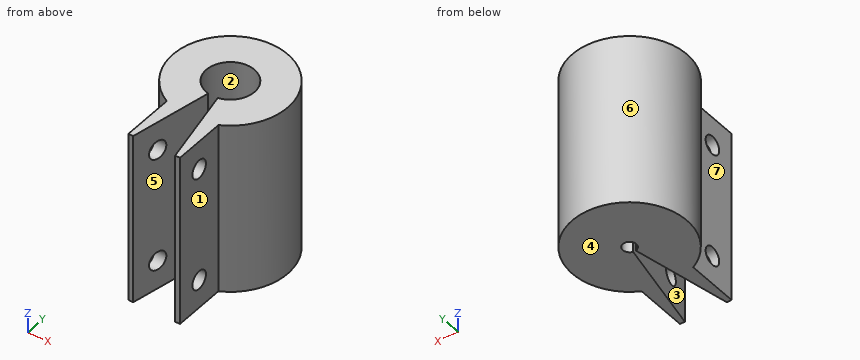
```python
from build123d import *

# Parameters (mm, degrees)
EXTRUDE_1_DEPTH     = 30
SKETCH_2_R          = 4.2
CUT_EXTRUDE_1_DEPTH = 15
SKETCH_3_R          = 1.175
CUT_EXTRUDE_2_DEPTH = 15
SKETCH_10_R         = 1.6
CUT_EXTRUDE_8_DEPTH = 38.871493237
CUT_EXTRUDE_9_DEPTH = 37.386810797


with BuildPart() as part:
    # ｽｹｯﾁ1 → ﾎﾞｽ - 押し出し1 (new body)
    with BuildSketch(Plane.XY):
        with BuildLine():
            Line((-4.5, -8.93028555), (-4.5, -18))
            Line((-4.5, -18), (4.5, -18))
            Line((4.5, -18), (4.5, -8.93028555))
            ThreePointArc((4.5, -8.93028555), (0, 10), (-4.5, -8.93028555))
        make_face()
    extrude(amount=EXTRUDE_1_DEPTH)

    # ｽｹｯﾁ2 → ｶｯﾄ - 押し出し1 (cut)
    with BuildSketch(Plane.XY.offset(30)):
        Circle(SKETCH_2_R)
    extrude(amount=-CUT_EXTRUDE_1_DEPTH, mode=Mode.SUBTRACT)

    # ｽｹｯﾁ3 → ｶｯﾄ - 押し出し2 (cut)
    with BuildSketch(Plane(origin=(0, 0, 0), x_dir=(-1, 0, 0), z_dir=(0, 0, -1))):
        Circle(SKETCH_3_R)
    extrude(amount=-CUT_EXTRUDE_2_DEPTH, mode=Mode.SUBTRACT)

    # ｽｹｯﾁ10 → ｶｯﾄ - 押し出し8 (cut, through all)
    with BuildSketch(Plane(origin=(4.5, 0, 0), x_dir=(0, 0, -1), z_dir=(1, 0, 0))):
        with Locations(Location((-25, -13.465142775, 0), (0, 0, 90))):
            Circle(SKETCH_10_R)
        with Locations(Location((-5, -13.465142775, 0), (0, 0, 90))):
            Circle(SKETCH_10_R)
    extrude(amount=-CUT_EXTRUDE_8_DEPTH, mode=Mode.SUBTRACT)

    # ｽｹｯﾁ4 → ｶｯﾄ - 押し出し9 (cut, through all)
    with BuildSketch(Plane.XY.offset(30)):
        with BuildLine():
            Line((-0.234043532, -1.151455003), (-3.658661061, -18))
            ThreePointArc((-3.658661061, -18), (0, -18.368064698), (3.658661061, -18))
            Line((3.658661061, -18), (0.234043532, -1.151455003))
            ThreePointArc((0.234043532, -1.151455003), (0, -1.175), (-0.234043532, -1.151455003))
        make_face()
    extrude(amount=-CUT_EXTRUDE_9_DEPTH, mode=Mode.SUBTRACT)


solid = part.part
```
The model under review builds one solid part; all positions refer to its coordinate system, in mm. Face numbers are marked on the shaded views. A direction names the side the tool comes from. Round coordinates to 2 decimals unless told otherwise and drop trailing zeros. Loops run counter-clockwise (first coordinate to the right, second up) from the corner with the lowest first, then second, coordinate; pieces in that order, holes last. Notation, with made-up numbers: (11, -12) -> (22, -12) arc R10 cw to (22, 4) -> close; hole circle Ø3 at (-6, -7). An arc over 180 degrees is marked (long way). Answer in a Markdown table with one row per item.
1) For pin 1 Ø10 at (y, z) = (-15.5, 20) entering from -X; pin 2 Ø6 at (x, y) = (-3, 6) entering from -Z; pin 3 Ø7.5 at (y, z) = (-13, 8.5) entering from +X; pin 4 Ø8 at (x, z) = (5, 21) entering from +Y, all flat-tipped, find the tip position at first contact; note any pin that passes through.
Taken from the geometry:
| item | result |
|---|---|
| pin 1 | stops at x = -4.5 |
| pin 2 | stops at z = 0 |
| pin 3 | stops at x = 4.5 |
| pin 4 | stops at y = 9.95 |
2) Draft analysis for pull direction X (two halves, no side actions). For the marked faces 5, 6 and 7, state which applies: pulls with the +X half, pulls with the -X half, needs draft (parallel to the pull), parting line crosses it, or undercut.
Taken from the geometry:
| item | result |
|---|---|
| face 5 | undercut |
| face 6 | parting line crosses it |
| face 7 | pulls with the -X half |
3) Consider section B-B, the plane z = 11.25. Write out the cut boundary in (x, y) (3 decimals).
Taken from the geometry:
| item | result |
|---|---|
| outline | (-4.5, -18) -> (-3.659, -18) -> (-0.234, -1.151) arc R1.175 cw (long way) to (0.234, -1.151) -> (3.659, -18) -> (4.5, -18) -> (4.5, -8.93) arc R10 ccw (long way) to (-4.5, -8.93) -> close |
4) Consider section C-C, the plane z = 25. Write out the cut boundary in (x, y), plus the area to 3 significant figures.
Taken from the geometry:
| item | result |
|---|---|
| outline | (-4.5, -18) -> (-3.66, -18) -> (-3.06, -15.07) -> (-4.5, -15.07) -> close; (-4.5, -11.87) -> (-2.41, -11.87) -> (-0.84, -4.12) arc R4.2 cw (long way) to (0.84, -4.12) -> (2.41, -11.87) -> (4.5, -11.87) -> (4.5, -8.93) arc R10 ccw (long way) to (-4.5, -8.93) -> close; (3.06, -15.07) -> (3.66, -18) -> (4.5, -18) -> (4.5, -15.07) -> close |
| area | 260 mm² |
5) Consider section D-D, the plane y = -7.5. Write out the cut boundary in (x, z), plus the area to 3 significant figures.
Taken from the geometry:
| item | result |
|---|---|
| outline | (-6.61, 0) -> (-1.52, 0) -> (-1.52, 30) -> (-6.61, 30) -> close; (1.52, 0) -> (6.61, 0) -> (6.61, 30) -> (1.52, 30) -> close |
| area | 305 mm² |
6) Tool access review of the marked faces 1, 2, 3 and 4: name each direction out of +Z, -Z, +X, -X, +Y, -Y from which nothing blocks a thin tool from reaching the whole face with its end or side.
Taken from the geometry:
| item | result |
|---|---|
| face 1 | +Z, -Z, +X, -Y |
| face 2 | +Z |
| face 3 | +Z, -Z, -Y |
| face 4 | -Z, +X, -X, +Y, -Y |
7) Wall thickness on line 1 along X through (y, z) = (0, 11.75) (3 decimals); line 2 along X through (y, z) = (-10, 12); line 3 along Z through (x, y) = (-2.75, 2.75): over which ranges is each line inside the solid? List them lowest first.
Taken from the geometry:
| item | result |
|---|---|
| line 1 | x = -10 to -1.175, 1.175 to 10 |
| line 2 | x = -4.5 to -2.03, 2.03 to 4.5 |
| line 3 | z = 0 to 15 |
8) Consider section A-A, the plane y = 0. Write out the cut boundary in (x, z) (3 decimals), plus the area to 3 significant figures.
Taken from the geometry:
| item | result |
|---|---|
| outline | (-10, 0) -> (-1.175, 0) -> (-1.175, 15) -> (-4.2, 15) -> (-4.2, 30) -> (-10, 30) -> close; (1.175, 0) -> (10, 0) -> (10, 30) -> (4.2, 30) -> (4.2, 15) -> (1.175, 15) -> close |
| area | 439 mm² |
